Autodesk Inventor part; units mm, degrees
ref_plane "YZ Plane" through (0, 0, 0) normal (1, 0, 0) x (0, 1, 0)
ref_plane "XZ Plane" through (0, 0, 0) normal (0, 1, 0) x (-1, 0, 0)
ref_plane "XY Plane" through (0, 0, 0) normal (0, 0, 1) x (1, 0, 0)
sketch "Sketch6" plane through (0, 0, 0) normal (0, 0, 1) x (1, 0, 0)
  circle A0 centre (0, 0) radius 72.5
  circle A1 centre (0, 0) radius 112.5
  dimension "d46" = 145
  dimension "d47" = 225
extrude "Plate1" add sketch "Sketch6" along normal blind 10
sketch "Sketch7" plane through (0, 0, 10) normal (0, 0, 1) x (1, 0, 0)
  circle A0 centre (0, 0) radius 81.5
  circle A1 centre (0, 0) radius 103.5
  dimension "d57" = 163
  dimension "d58" = 207
extrude "Extrusion5" cut sketch "Sketch7" against normal blind 3.5
sketch "Sketch8" plane through (0, 0, 0) normal (0, 0, -1) x (-1, 0, 0)
  circle A0 centre (0, 92.5) radius 5.5
  circle A1 centre (0, 0) radius 92.5 construction
  dimension "d51" = 185
  dimension "d50" = 11
extrude "Extrusion6" cut sketch "Sketch8" along normal through all both and the other way through all
pattern_circular "Circular Pattern3" count 6 over 360 about axis through (0, 0, 0) along (0, 0, 1) of "Extrusion6"
equation "\"d47\" = back_steel_circle_диам_центров + back_steel_circle_ширина_кольца"
equation "\"d51\" = back_steel_circle_диам_центров"
equation "\"d45\" = Thickness"
equation "\"BendReliefDepth\" = 0.5 * Thickness"
properties part number "NVPH-322 joint HDPE ring"
Design review of the part built by this model. Coordinates are the model's own, in mm. A direction names the side the tool comes from. Give positions to 0.01 mm unless a question says otherwise; leave off trailing zeros. Loops run counter-clockwise (first coordinate to the right, second up) from the corner with the lowest first, then second, coordinate; pieces in that order, holes last. Notation, with made-up numbers: (-7.5, 46) -> (21.5, 46) arc R23 cw to (21.5, 77) -> close; hole circle Ø3 at (26.25, 20). An arc over 180 degrees is marked (long way). One line per question, with ' | ' between items. Start each with the question number.
(1) Insertion check: P1, Ø1, axis at x = -88.5, z = 4, coming from the -Y side; P2, Ø1.5, axis at y = -50, z = 5, coming from the -X side; P3, Ø5, axis at x = 72.5, z = 1, coming from the -Y side; P4, Ø6.5, axis at x = 0, y = -92.5, coming from the -Z side. Each pin has a flat end and moves straight along its axis. Give the tip position at first contact, or say it passes through.
(2) We need section D-D (y = -47). State the section outline as (x, z) points.
(3) We need section B-B (z = 8.5). State the section outline as (x, y) points.
(4) For line 1 (Y direction, x = 0, z = 9.05); line 2 (Y direction, x = 0, z = 5); line 3 (X direction, y = -35.5, z = 7), list the stretches that pass through material, from the lowest coordinate up.
(5) Draft analysis for pull direction X (two halves, no side actions). For faces 3 (the face through (-112.39, -4.95, 4.93)), 4 (the face through (-0.716, -97.953, 3.204)), 5 (the face through (73, 2, 0)), state which applies: +X half, -X half, draft (parallel to the pull), parting line (faces both ways), or undercut.
(6) We need section A-A (y = 0). State the section outline as (x, z) points.
(7) We need section C-C (x = 0). State the section outline as (y, z) points, and give its area (3 significant figures).
(8) For faces 1 (the face through (75.285, -31.215, 8.274)), 2 (the face through (-55, -48, 10)), list the 3-axis set-ups (+Z, -Z, +X, -X, +Y, -Y) from which the entire face can be reached by the end or side of a thin tool; tool diameter is ignored.
The answers:
1) P1: stops at y = -70.09 | P2: stops at x = -101.15 | P3: stops at y = -88.07 | P4: passes through
2) outline: (-102.21, 0) -> (-85.56, 0) -> (-85.56, 6.5) -> (-92.21, 6.5) -> (-92.21, 10) -> (-102.21, 10) -> close; (-74.66, 0) -> (-55.2, 0) -> (-55.2, 10) -> (-66.58, 10) -> (-66.58, 6.5) -> (-74.66, 6.5) -> close; (55.2, 0) -> (74.66, 0) -> (74.66, 6.5) -> (66.58, 6.5) -> (66.58, 10) -> (55.2, 10) -> close; (85.56, 0) -> (102.21, 0) -> (102.21, 10) -> (92.21, 10) -> (92.21, 6.5) -> (85.56, 6.5) -> close
3) outline: circle Ø225 at (0, 0); circle Ø163 at (0, 0); hole circle Ø207 at (0, 0); hole circle Ø145 at (0, 0)
4) line 1: y = -112.5 to -103.5, -81.5 to -72.5, 72.5 to 81.5, 103.5 to 112.5 | line 2: y = -112.5 to -98, -87 to -72.5, 72.5 to 87, 98 to 112.5 | line 3: x = -106.75 to -97.22, -73.36 to -63.21, 63.21 to 73.36, 97.22 to 106.75
5) face 3: parting line | face 4: undercut | face 5: draft
6) outline: (-112.5, 0) -> (-72.5, 0) -> (-72.5, 10) -> (-81.5, 10) -> (-81.5, 6.5) -> (-103.5, 6.5) -> (-103.5, 10) -> (-112.5, 10) -> close; (72.5, 0) -> (112.5, 0) -> (112.5, 10) -> (103.5, 10) -> (103.5, 6.5) -> (81.5, 6.5) -> (81.5, 10) -> (72.5, 10) -> close
7) outline: (-112.5, 0) -> (-98, 0) -> (-98, 6.5) -> (-103.5, 6.5) -> (-103.5, 10) -> (-112.5, 10) -> close; (-87, 0) -> (-72.5, 0) -> (-72.5, 10) -> (-81.5, 10) -> (-81.5, 6.5) -> (-87, 6.5) -> close; (72.5, 0) -> (87, 0) -> (87, 6.5) -> (81.5, 6.5) -> (81.5, 10) -> (72.5, 10) -> close; (98, 0) -> (112.5, 0) -> (112.5, 10) -> (103.5, 10) -> (103.5, 6.5) -> (98, 6.5) -> close | area: 503 mm^2
8) face 1: +Z | face 2: +Z, +X, -X, +Y, -Y
